```python
from build123d import *

# Parameters (mm, degrees)
SKETCH1_R             = 20
SKETCH1_R_2           = 15
BOSS_EXTRUDE1_DEPTH   = 15
SKETCH1_R_3           = 40
SKETCH1_R_4           = 16
BOSS_EXTRUDE1_2_DEPTH = 15
BOSS_EXTRUDE1_3_DEPTH = 15
SKETCH1_3_R           = 15
BOSS_EXTRUDE2_DEPTH   = 7.5


with BuildPart() as part:
    # Sketch1 → Boss-Extrude1 (new, symmetric)
    with BuildSketch(Plane.XY):
        with Locations((-70, 0)):
            Circle(SKETCH1_R)
        with Locations((-70, 0)):
            Circle(SKETCH1_R_2, mode=Mode.SUBTRACT)
    extrude(amount=BOSS_EXTRUDE1_DEPTH, both=True)



with BuildPart() as body_2:
    # Sketch1 → Boss-Extrude1 2 (new, symmetric)
    with BuildSketch(Plane.XY):
        Circle(SKETCH1_R_3)
        Circle(SKETCH1_R_4, mode=Mode.SUBTRACT)
        with BuildLine():
            ThreePointArc((29.090759323, -13.331456111), (32, 0), (29.090759323, 13.331456111))
            Line((29.090759323, 13.331456111), (19.5, 7.794228634))
            ThreePointArc((19.5, 7.794228634), (21, 0), (19.5, -7.794228634))
            Line((19.5, -7.794228634), (29.090759323, -13.331456111))
        make_face(mode=Mode.SUBTRACT)
        with BuildLine():
            ThreePointArc((3, -31.859064644), (16, -27.712812921), (26.090759323, -18.527608533))
            Line((26.090759323, -18.527608533), (16.5, -12.990381057))
            ThreePointArc((16.5, -12.990381057), (10.5, -18.186533479), (3, -20.784609691))
            Line((3, -20.784609691), (3, -31.859064644))
        make_face(mode=Mode.SUBTRACT)
        with BuildLine():
            ThreePointArc((-26.090759323, -18.527608533), (-16, -27.712812921), (-3, -31.859064644))
            Line((-3, -31.859064644), (-3, -20.784609691))
            ThreePointArc((-3, -20.784609691), (-10.5, -18.186533479), (-16.5, -12.990381057))
            Line((-16.5, -12.990381057), (-26.090759323, -18.527608533))
        make_face(mode=Mode.SUBTRACT)
        with BuildLine():
            ThreePointArc((-29.090759323, 13.331456111), (-32, 0), (-29.090759323, -13.331456111))
            Line((-29.090759323, -13.331456111), (-19.5, -7.794228634))
            ThreePointArc((-19.5, -7.794228634), (-21, 0), (-19.5, 7.794228634))
            Line((-19.5, 7.794228634), (-29.090759323, 13.331456111))
        make_face(mode=Mode.SUBTRACT)
        with BuildLine():
            Line((16.5, 12.990381057), (26.090759323, 18.527608533))
            ThreePointArc((26.090759323, 18.527608533), (16, 27.712812921), (3, 31.859064644))
            Line((3, 31.859064644), (3, 20.784609691))
            ThreePointArc((3, 20.784609691), (10.5, 18.186533479), (16.5, 12.990381057))
        make_face(mode=Mode.SUBTRACT)
        with BuildLine():
            Line((-3, 20.784609691), (-3, 31.859064644))
            ThreePointArc((-3, 31.859064644), (-16, 27.712812921), (-26.090759323, 18.527608533))
            Line((-26.090759323, 18.527608533), (-16.5, 12.990381057))
            ThreePointArc((-16.5, 12.990381057), (-10.5, 18.186533479), (-3, 20.784609691))
        make_face(mode=Mode.SUBTRACT)
    extrude(amount=BOSS_EXTRUDE1_2_DEPTH, both=True)


with BuildPart() as body_3:
    # Sketch1 → Boss-Extrude1 3 (new, symmetric)
    with BuildSketch(Plane.XY):
        with Locations((70, 0)):
            Circle(SKETCH1_R)
        with Locations((70, 0)):
            Circle(SKETCH1_R_2, mode=Mode.SUBTRACT)
    extrude(amount=BOSS_EXTRUDE1_3_DEPTH, both=True)


with BuildPart() as part_1:
    add(part.part)

    add(body_2.part)  # Boss-Extrude2 merges body 2

    add(body_3.part)  # Boss-Extrude2 merges body 3
    # Sketch1_3 → Boss-Extrude2 (add, symmetric)
    # profile 1 of 2: a face of its own
    with BuildSketch(Plane.XY):
        with BuildLine():
            ThreePointArc((-50, 0), (-66.95253237, -19.766460003), (-89.071294105, -6.023764702))
            Line((-89.071294105, -6.023764702), (-70.02485881, -66.324952937))
            ThreePointArc((-70.02485881, -66.324952937), (-46.6282273, -80.727545655), (-29.002885891, -59.651863383))
            ThreePointArc((-29.002885891, -59.651863383), (-22.168588856, -44.262528341), (-6.003756239, -39.546869801))
            ThreePointArc((-6.003756239, -39.546869801), (-40, 0), (-6.003756239, 39.546869801))
            ThreePointArc((-6.003756239, 39.546869801), (-22.168588856, 44.262528341), (-29.002885891, 59.651863383))
            ThreePointArc((-29.002885891, 59.651863383), (-46.6282273, 80.727545655), (-70.02485881, 66.324952937))
            Line((-70.02485881, 66.324952937), (-89.071294105, 6.023764702))
            ThreePointArc((-89.071294105, 6.023764702), (-66.95253237, 19.766460003), (-50, 0))
        make_face()
        with Locations((-50, -60)):
            Circle(SKETCH1_3_R, mode=Mode.SUBTRACT)
        with Locations((-50, 60)):
            Circle(SKETCH1_3_R, mode=Mode.SUBTRACT)
    # profile 2 of 2: a face of its own
    with BuildSketch(Plane.XY):
        with BuildLine():
            ThreePointArc((40, 0), (30.332740146, -26.075369129), (6.003756239, -39.546869801))
            ThreePointArc((6.003756239, -39.546869801), (22.168588856, -44.262528341), (29.002885891, -59.651863383))
            ThreePointArc((29.002885891, -59.651863383), (46.6282273, -80.727545655), (70.02485881, -66.324952937))
            Line((70.02485881, -66.324952937), (89.071294105, -6.023764702))
            ThreePointArc((89.071294105, -6.023764702), (50, 0), (89.071294105, 6.023764702))
            Line((89.071294105, 6.023764702), (70.02485881, 66.324952937))
            ThreePointArc((70.02485881, 66.324952937), (46.6282273, 80.727545655), (29.002885891, 59.651863383))
            ThreePointArc((29.002885891, 59.651863383), (22.168588856, 44.262528341), (6.003756239, 39.546869801))
            ThreePointArc((6.003756239, 39.546869801), (30.332740146, 26.075369129), (40, 0))
        make_face()
        with Locations((50, -60)):
            Circle(SKETCH1_3_R, mode=Mode.SUBTRACT)
        with Locations((50, 60)):
            Circle(SKETCH1_3_R, mode=Mode.SUBTRACT)
    extrude(amount=BOSS_EXTRUDE2_DEPTH, both=True)


solid = part_1.part
```
Check sheet for the modelled part. Datum: model origin and axes. Units: mm. A direction names the side the tool comes from. Round coordinates to 2 decimals unless told otherwise and drop trailing zeros. Order: outer loops, then holes, each group sorted by start corner. A loop starts at its lowest first (then second) coordinate and runs counter-clockwise, first axis right, second up.
1) Scan lines: line 1 (X direction, y = 0.5, z = 3.5); line 2 (Y direction, x = 50, z = -5.5); line 3 (Y direction, x = 56.5, z = 7). Record each from-to range of solid material in increasing order.
2) Section check C-C (y = 51). Record the boundary of the cut face in (x, z).
3) Mould release check, pull along X, two halves, no side actions. Record for faces 1 (the flat face through (-3, 26, 0)), 2 (the cylindrical face through (-89.98, 0.88, 0.21)), 3 (the flat face through (-67, 15, 15)): +X half, -X half, draft (parallel to the pull), parting line (faces both ways), or undercut.
4) Go/stop test with flat-tipped pins: pin 1 Ø6 at (y, z) = (7, -9) entering from -X; pin 2 Ø3.5 at (y, z) = (27.5, 0.5) entering from +X; pin 3 Ø12 at (y, z) = (-24.5, 6) entering from +X. Record where each tip stops, or that it passes through.
5) Section check B-B (y = 23.5). Record the boundary of the cut face in (x, z).
6) Section check D-D (x = 76). Record the boundary of the cut face in (y, z), and give its area (3 significant figures).
7) Tool access check on faces 4 (the cylindrical face through (-5.21, 39.66, 0.21)), 5 (the flat face through (47, 6, 7.5)), 6 (the flat face through (47, 6, -7.5)), 7 (the flat face through (-21.363, 15.798, 0.21)). Record the directions out of +Z, -Z, +X, -X, +Y, -Y that give a thin tool (end or side, any length) a straight path to the whole face; none if there is none.
8) Section check A-A (x = 0). Record the boundary of the cut face in (y, z).
Result:
1. line 1: x = -89.99 to -84.99, -55.01 to -32, -20.99 to -15.99, 15.99 to 20.99, 32 to 55.01, 84.99 to 89.99
1. line 2: y = -81 to -75, -45 to 45, 75 to 81
1. line 3: y = -79.97 to -73.52, -46.48 to -6.54, 6.54 to 46.48, 73.52 to 79.97
2. outline: (-74.87, -7.5) - (-62, -7.5) - (-62, 7.5) - (-74.87, 7.5) - close; (-38, -7.5) - (-27.19, -7.5) - (-27.19, 7.5) - (-38, 7.5) - close; (27.19, -7.5) - (38, -7.5) - (38, 7.5) - (27.19, 7.5) - close; (62, -7.5) - (74.87, -7.5) - (74.87, 7.5) - (62, 7.5) - close
3. face 1: undercut
3. face 2: undercut
3. face 3: draft
4. pin 1: stops at x = -89.6
4. pin 2: stops at x = 82.84
4. pin 3: stops at x = 85.13
5. outline: (-83.55, -7.5) - (-32.37, -7.5) - (-32.37, -15) - (-21.72, -15) - (-21.72, 15) - (-32.37, 15) - (-32.37, 7.5) - (-83.55, 7.5) - close; (-3, -15) - (3, -15) - (3, 15) - (-3, 15) - close; (21.72, -15) - (32.37, -15) - (32.37, -7.5) - (83.55, -7.5) - (83.55, 7.5) - (32.37, 7.5) - (32.37, 15) - (21.72, 15) - close
6. outline: (-47.41, -7.5) - (-19.08, -7.5) - (-19.08, -15) - (-13.75, -15) - (-13.75, 15) - (-19.08, 15) - (-19.08, 7.5) - (-47.41, 7.5) - close; (13.75, -15) - (19.08, -15) - (19.08, -7.5) - (47.41, -7.5) - (47.41, 7.5) - (19.08, 7.5) - (19.08, 15) - (13.75, 15) - close
6. area: 1,170 mm2
7. face 4: none
7. face 5: +Z
7. face 6: -Z
7. face 7: +Z, -Z
8. outline: (-40, -15) - (-16, -15) - (-16, 15) - (-40, 15) - close; (16, -15) - (40, -15) - (40, 15) - (16, 15) - close
